```python
from build123d import *

# Parameters (mm, degrees)
BOSS_EXTRUDE1_DEPTH = 2.54
SKETCH4_W           = 36.068
SKETCH4_H           = 35.56
BOSS_EXTRUDE2_DEPTH = 2.54
SKETCH5_W           = 19.05
SKETCH5_H           = 25.4
CUT_EXTRUDE1_DEPTH  = 44.540075149
SKETCH7_R           = 0.762
BOSS_EXTRUDE3_DEPTH = 7.62
SKETCH9_W           = 12.7
SKETCH9_H           = 25.4
SKETCH9_R           = 1.524
BOSS_EXTRUDE4_DEPTH = 2.54


with BuildPart() as part:
    # Sketch1 → Boss-Extrude1 (new body)
    with BuildSketch(Plane(origin=(0, 0, 0), x_dir=(1, 0, 0), z_dir=(0, 1, 0))):
        Polygon((-5.08, 30.48), (30.988, 30.48), (30.988, -5.08), (21.844, -5.08), (21.844, 0), (25.908, 0), (25.908, 25.4), (0, 25.4), (0, 0), (4.064, 0), (4.064, -5.08), (-5.08, -5.08), align=None)
    extrude(amount=BOSS_EXTRUDE1_DEPTH)

    # Sketch4 → Boss-Extrude2 (add)
    with BuildSketch(Plane(origin=(0, 2.54, 0), x_dir=(1, 0, 0), z_dir=(0, 1, 0))):
        with Locations((12.954, 12.7)):
            Rectangle(SKETCH4_W, SKETCH4_H)
    extrude(amount=BOSS_EXTRUDE2_DEPTH)

    # Sketch5 → Cut-Extrude1 (cut, through all)
    with BuildSketch(Plane.XZ.offset(-2.54)):
        with Locations((12.954, -12.7)):
            Rectangle(SKETCH5_W, SKETCH5_H)
    extrude(amount=-CUT_EXTRUDE1_DEPTH, mode=Mode.SUBTRACT)

    # Sketch7 → Boss-Extrude3 (add)
    with BuildSketch(Plane.XZ.offset(-2.54)):
        with Locations(Location((2.159, -10.16, 0), (0, 0, 90))):
            Circle(SKETCH7_R)
        with Locations(Location((2.159, -22.86, 0), (0, 0, 90))):
            Circle(SKETCH7_R)
        with Locations(Location((23.749, -10.16, 0), (0, 0, 90))):
            Circle(SKETCH7_R)
        with Locations(Location((23.749, -22.86, 0), (0, 0, 90))):
            Circle(SKETCH7_R)
    extrude(amount=BOSS_EXTRUDE3_DEPTH)

    # Sketch9 → Boss-Extrude4 (add)
    with BuildSketch(Plane(origin=(30.988, 0, 0), x_dir=(0, 0, -1), z_dir=(1, 0, 0))):
        with Locations((1.27, -7.62)):
            Rectangle(SKETCH9_W, SKETCH9_H)
        with Locations((1.27, -5.08)):
            Circle(SKETCH9_R, mode=Mode.SUBTRACT)
        with Locations((1.27, -15.24)):
            Circle(SKETCH9_R, mode=Mode.SUBTRACT)
    extrude(amount=BOSS_EXTRUDE4_DEPTH)


solid = part.part
```
For this review, take the finished solid that the model builds, in its own axes (mm). A direction names the side the tool comes from. Coordinates: 2 decimals unless noted, no trailing zeros. Write each loop counter-clockwise with the first axis right and the second up, starting at its lowest first coordinate (ties: lowest second). Pieces come first, ordered by that corner, then holes.
(1) Add section A-A on y = -15.24. Give the boundary of the cut face in (x, z).
(2) For pin 1 Ø3 at (y, z) = (1, -18.5) entering from +X; pin 2 Ø1.3 at (x, y) = (31.5, -12) entering from -Z; pin 3 Ø1.2 at (x, z) = (2, -10.5) entering from -Y, all flat-tipped, find the tip position at first contact; note any pin that passes through.
(3) Tool access review of faces 1 (the face through (13, 3, -25.4)), 2 (the face through (4.064, 1, 3)), 3 (the face through (30.988, -10, -1)): name each direction out of +Z, -Z, +X, -X, +Y, -Y from which nothing blocks a thin tool from reaching the whole face with its end or side.
(4) Wall thickness on probe 1 along Y at (x, z) = (32.15, -1.27); probe 2 along Y at (x, z) = (32, -1); probe 3 along X at (y, z) = (0.5, -11): over which ranges is each line inside the solid? List them lowest first.
(5) Add section B-B on z = -1.27. Give the boundary of the cut face in (x, y).
(6) Add section D-D on z = -11.5. Give the boundary of the cut face in (x, y).
(7) The part is to be moulded in two halves that separate along Z. For faces 4 (the face through (23.106, -1.217, -22.45)), 5 (the face through (23, 5.08, -12)), 6 (the face through (13, 3, -30.48)), say which applies: +Z half, -Z half, draft (parallel to the pull), parting line (faces both ways), or undercut.
(8) Add section C-C on x = 16. Give the boundary of the cut face in (y, z), then the cut area to 3 significant figures.
Answer sheet:
1. outline: (30.99, -7.62) - (33.53, -7.62) - (33.53, -2.79) - (30.99, -2.79) - close; (30.99, 0.25) - (33.53, 0.25) - (33.53, 5.08) - (30.99, 5.08) - close
2. pin 1: stops at x = 30.99
2. pin 2: stops at z = -7.62
2. pin 3: stops at y = -5.08
3. face 1: -Y
3. face 2: +Z, -Y
3. face 3: +Z, -Z, -X, -Y
4. probe 1: y = -20.32 to -16.76, -13.72 to -6.6, -3.56 to 5.08
4. probe 2: y = -20.32 to -16.74, -13.74 to -6.58, -3.58 to 5.08
4. probe 3: x = -5.08 to 0, 25.91 to 30.99
5. outline: (-5.08, 0) - (0, 0) - (0, 2.54) - (3.43, 2.54) - (3.43, 5.08) - (-5.08, 5.08) - close; (22.48, 2.54) - (25.91, 2.54) - (25.91, 0) - (30.99, 0) - (30.99, -3.56) - (33.53, -3.56) - (33.53, 5.08) - (22.48, 5.08) - close; (30.99, -20.32) - (33.53, -20.32) - (33.53, -16.76) - (30.99, -16.76) - close; (30.99, -13.72) - (33.53, -13.72) - (33.53, -6.6) - (30.99, -6.6) - close
6. outline: (-5.08, 0) - (0, 0) - (0, 2.54) - (3.43, 2.54) - (3.43, 5.08) - (-5.08, 5.08) - close; (22.48, 2.54) - (25.91, 2.54) - (25.91, 0) - (30.99, 0) - (30.99, 5.08) - (22.48, 5.08) - close
7. face 4: undercut
7. face 5: draft
7. face 6: -Z half
8. outline: (0, -30.48) - (5.08, -30.48) - (5.08, -25.4) - (0, -25.4) - close; (2.54, 0) - (5.08, 0) - (5.08, 5.08) - (2.54, 5.08) - close
8. area: 38.7 mm2
